```python
from build123d import *

# Parameters (mm, degrees)
BOSS_EXTRUDE1_DEPTH = 30


with BuildPart() as part:
    # Sketch4 → Boss-Extrude1 (new body, symmetric)
    with BuildSketch(Plane.XY):
        with BuildLine():
            Line((4.8, -20), (17.2, -20))
            ThreePointArc((17.2, -20), (19.179898987, -19.179898987), (20, -17.2))
            Line((20, -17.2), (20, -4.8))
            ThreePointArc((20, -4.8), (19.765685425, -4.234314575), (19.2, -4))
            Line((19.2, -4), (16.190663761, -4))
            ThreePointArc((16.190663761, -4), (15.624978336, -4.234314575), (15.390663761, -4.8))
            Line((15.390663761, -4.8), (15.390663761, -10.2))
            ThreePointArc((15.390663761, -10.2), (14.896810507, -10.939103626), (14.024978336, -10.765685425))
            Line((14.024978336, -10.765685425), (9.40588745, -6.146594539))
            ThreePointArc((9.40588745, -6.146594539), (8.365378244, -4.589362465), (8, -2.752481989))
            Line((8, -2.752481989), (8, 0))
            Line((8, 0), (3.5, 0))
            ThreePointArc((3.5, 0), (2.474873734, -2.474873734), (0, -3.5))
            Line((0, -3.5), (0, -8))
            Line((0, -8), (2.752481989, -8))
            ThreePointArc((2.752481989, -8), (4.589362465, -8.365378244), (6.146594539, -9.40588745))
            Line((6.146594539, -9.40588745), (10.765685425, -14.024978336))
            ThreePointArc((10.765685425, -14.024978336), (10.939103626, -14.896810507), (10.2, -15.390663761))
            Line((10.2, -15.390663761), (4.8, -15.390663761))
            ThreePointArc((4.8, -15.390663761), (4.234314575, -15.624978336), (4, -16.190663761))
            Line((4, -16.190663761), (4, -19.2))
            ThreePointArc((4, -19.2), (4.234314575, -19.765685425), (4.8, -20))
        make_face()
    extrude(amount=BOSS_EXTRUDE1_DEPTH, both=True)

    # Mirror1: part across plane


with BuildPart() as part_1:
    add(part.part)
    add(part.part.mirror(Plane(origin=(0, 0, 0), x_dir=(0, 0, 1), z_dir=(1, 0, 0))))

    # Mirror2: part across plane


with BuildPart() as part_2:
    add(part_1.part)
    add(part_1.part.mirror(Plane.ZX))


solid = part_2.part
```
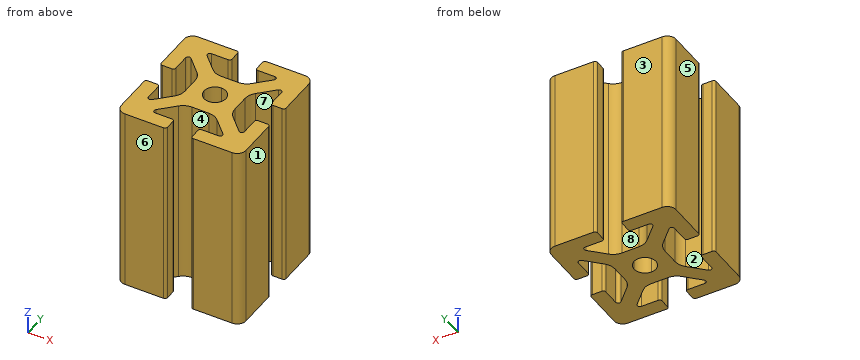
Here's how the part is built. I have some questions about the finished solid (model axes, mm). Face numbers are marked on the shaded views. A direction names the side the tool comes from. Coordinates: 2 decimals unless noted, no trailing zeros. Loops run counter-clockwise (first coordinate to the right, second up) from the corner with the lowest first, then second, coordinate; pieces in that order, holes last. Notation, with made-up numbers: M -16.5,-7.75 L 36.5,-7.75 A14 ccw 36.5,7.25 Z; hole C 6,-20 d8. An arc over 180 degrees is marked long. One line per item, written item: value.
1. Thinking about a two-plate mould opening in Y: for the marked faces 1, 2 and 3, which applies, +Y half, -Y half, draft (parallel to the pull), parting line (faces both ways), or undercut?
Geometry says:
face 1: draft
face 2: undercut
face 3: +Y half
2. Will these pins go through, and if not, where does the flat tip stop? pin 1 Ø3 at (x, z) = (-1.5, 0.5) entering from +Y; pin 2 Ø1 at (y, z) = (-3, 3) entering from +X; pin 3 Ø4.5 at (x, z) = (-0.5, 4.5) entering from -Y.
Geometry says:
pin 1: stops at y = 8.01
pin 2: stops at x = 8.06
pin 3: stops at y = -8
3. Imagine slicing it at A-A (x = 12.5). List the corners of the cut face in (y, z) for me.
Geometry says:
outline: M -20,-30 L -9.24,-30 L -9.24,30 L -20,30 Z; M 9.24,-30 L 20,-30 L 20,30 L 9.24,30 Z
4. Imagine slicing it at B-B (y = -7). List the corners of the cut face in (x, z) for me.
Geometry says:
outline: M -20,-30 L -15.39,-30 L -15.39,30 L -20,30 Z; M -10.26,-30 L 10.26,-30 L 10.26,30 L -10.26,30 Z; M 15.39,-30 L 20,-30 L 20,30 L 15.39,30 Z
5. Please list where these lines run through material, in increasing order: probe 1 along X at (y, z) = (7.5, -6); probe 2 along X at (y, z) = (-9, 10).
Geometry says:
probe 1: x = -20 to -15.39, -10.76 to 10.76, 15.39 to 20
probe 2: x = -20 to -15.39, -12.26 to -5.69, 5.69 to 12.26, 15.39 to 20
6. On a 3-axis mill with a long thin cutter (end or side, diameter ignored), from which of +Z, -Z, +X, -X, +Y, -Y can I reach the whole of each face in a straight line? I mean the marked faces 4, 5, 6, 7 and 8. Say none if no direction works.
Geometry says:
face 4: +Z, -Z, -Y
face 5: +Z, -Z, -X, +Y, -Y
face 6: +Z, -Z, +X, -X, -Y
face 7: +Z, -Z
face 8: +Z, -Z, +Y
